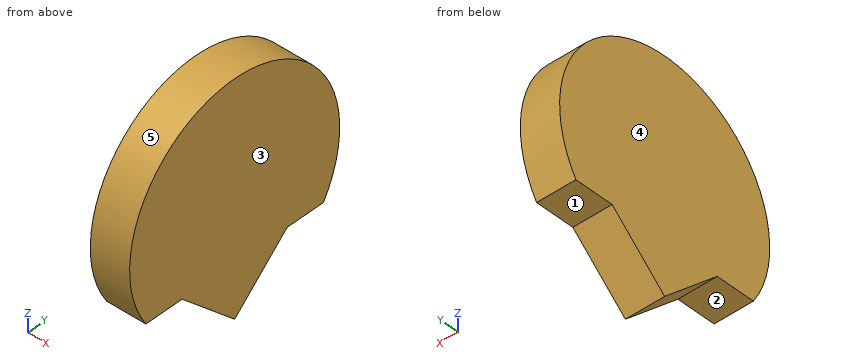
```python
from build123d import *

# Parameters (mm, degrees)
PAD008_DEPTH = 6.9


with BuildPart() as part:
    # Sketch018 → Pad008 (new body)
    with BuildSketch(Plane.YZ.offset(37.9)):
        with BuildLine():
            ThreePointArc((216.953369, 20.01), (200.05, 50.7), (183.146631, 20.01))
            Line((183.146631, 20.01), (190.05, 20.01))
            Line((190.05, 20.01), (200.05, 10.7))
            Line((210.05, 20.01), (200.05, 10.7))
            Line((216.953369, 20.01), (210.05, 20.01))
        make_face()
    extrude(amount=PAD008_DEPTH)


solid = part.part
```
Source: CAD feature listing. Evaluate the final solid. Frame: model axes, mm. Face numbers are marked on the shaded views. A direction names the side the tool comes from. Coordinates: 2 decimals unless noted, no trailing zeros. Loops run counter-clockwise (first coordinate to the right, second up) from the corner with the lowest first, then second, coordinate; pieces in that order, holes last. Notation, with made-up numbers: (-14.75, -22) - (19.25, -22) arc R25 ccw to (19.25, 14) - close; hole circle Ø9 at (64.5, 67). An arc over 180 degrees is marked (long way). Answer as CSV lines item,"result".
1. Reachability of the marked faces 1 and 2 from +Z, -Z, +X, -X, +Y, -Y: full face, straight path, thin tool, end or side. Return the list, or none.
Established:
face 1,"-Z, +X, -X, +Y"
face 2,"-Z, +X, -X, -Y"
2. Mould query, pull axis X, two halves, no side actions, for the marked faces 3, 4 and 5. Classes: released by +X, released by -X, zero draft, split by the parting line, or undercut.
Established:
face 3,"released by +X"
face 4,"released by -X"
face 5,"zero draft"
3. Section B-B (y = 191). Return loops of the section in (x, z).
Established:
outline,"(37.9, 19.13) - (44.8, 19.13) - (44.8, 48.54) - (37.9, 48.54) - close"
4. Section A-A (x = 42.75). Return loops of the section in (y, z).
Established:
outline,"(183.15, 20.01) - (190.05, 20.01) - (200.05, 10.7) - (210.05, 20.01) - (216.95, 20.01) arc R20 ccw (long way) to start"
5. Section C-C (z = 42.5). Return loops of the section in (x, y).
Established:
outline,"(37.9, 183.9) - (44.8, 183.9) - (44.8, 216.2) - (37.9, 216.2) - close"
6. Ray query, line 1 (Y direction, x = 44, z = 33); line 2 (Z direction, x = 39.75, y = 215.5); line 3 (Z direction, x = 43, y = 211). Return the intervals inside material, ascending.
Established:
line 1,"y = 180.18 to 219.92"
line 2,"z = 20.01 to 43.4"
line 3,"z = 20.01 to 47.44"
7. Contact query for flat-ended pins moving along their axis: pin 1 (1 mm diameter, centred on x = 43, z = 36, fed in from +Y); pin 2 (2 mm diameter, centred on x = 42.5, y = 186, fed in from -Z); pin 3 (4 mm diameter, centred on x = 43, y = 194, fed in from -Z). Output: stop coordinate, or through.
Established:
pin 1,"stops at y = 219.47"
pin 2,"stops at z = 20.01"
pin 3,"stops at z = 14.47"
